Work out the finished part from the listing and answer in its coordinate system (mm). A direction names the side the tool comes from. Give positions to 0.01 mm unless a question says otherwise; leave off trailing zeros. Write each loop counter-clockwise with the first axis right and the second up, starting at its lowest first coordinate (ties: lowest second). Pieces come first, ordered by that corner, then holes. Notation, with made-up numbers: (52, -14.75) -> (57, -14.75) arc R30 ccw to (57, 24.25) -> close; hole circle Ø10 at (27.5, -5.5). An arc over 180 degrees is marked (long way). Use a Markdown table: item, result. Add a question column.
Q1. Section C-C, the plane y = 18.5 is taken. Give the vertices of the cut face in (x, z), plus the area to 3 significant figures.
Q2. Section B-B, the plane y = 33 is taken. Give the vertices of the cut face in (x, z), plus the area to 3 significant figures.
Q3. For a pull along X with two mould halves and no side action, classify faces 5 (the face through (5.4, 31.75, 0.1)), 6 (the face through (-1, 12.7, 0)), 7 (the face through (4.89, 35, 0)) as pulls with the +X half, pulls with the -X half, needs draft (parallel to the pull), parting line crosses it, or undercut.
Q4. Section A-A, the plane y = 9.5 is taken. Give the vertices of the cut face in (x, z).
Q5. Consider line 1 (Y direction, x = 7.45, z = 0); line 2 (Y direction, x = 2.75, z = 3.5); line 3 (Z direction, x = 8.45, y = 6.35). Determine where each line is inside the solid, lowest interval first.
Q6. Each of these flat-tipped pins is pushed along its axis until it touches: pin 1 Ø1.5 at (x, z) = (7, 3.5) entering from +Y; pin 2 Ø0.7 at (x, z) = (5.5, 2) entering from +Y; pin 3 Ø1 at (x, y) = (1, 18) entering from -Z; pin 4 Ø1.5 at (y, z) = (33.5, -7.5) entering from -X. Where does it stop, or does it pass through?
Q7. For faces 1 (the face through (-6.233, 28.717, 0.818)), 2 (the face through (7.14, 7.53, -0.15)), 3 (the face through (0, 38.1, 0)), 4 (the face through (4.89, 8, 0)), determine the directions among +Z, -Z, +X, -X, +Y, -Y from which every point of the face is accessible in a straight line to the end or side of a thin tool.
from build123d import *

# Parameters (mm, degrees)
SKETCH1_R           = 6.2865
BASE_EXTRUDE_DEPTH  = 38.1
SKETCH3_R           = 9.4615
BOSS_EXTRUDE1_DEPTH = 15.875
CUT_EXTRUDE1_DEPTH  = 12.7
FILLET1_R           = 4.7625
FILLET2_R           = 4.7625
SKETCH5_R           = 1.190625
CUT_EXTRUDE2_DEPTH  = 42.798101456
CUT_EXTRUDE3_START  = -6.35
CUT_EXTRUDE3_DEPTH  = 6.35
CHAMFER1_SIZE       = 0.79375


with BuildPart() as part:
    # Sketch1 → Base-Extrude (new body)
    with BuildSketch(Plane(origin=(0, 0, 0), x_dir=(-1, 0, 0), z_dir=(0, 1, 0))):
        with Locations(Location((0, 0, 0), (0, 0, 270))):
            Circle(SKETCH1_R)
    extrude(amount=BASE_EXTRUDE_DEPTH)

    # Sketch3 → Boss-Extrude1 (add)
    with BuildSketch(Plane(origin=(0, 0, 0), x_dir=(-1, 0, 0), z_dir=(0, 1, 0))):
        with Locations(Location((0, 0, 0), (0, 0, 90))):
            Circle(SKETCH3_R)
    extrude(amount=BOSS_EXTRUDE1_DEPTH)

    # Sketch4 → Cut-Extrude1 (cut)
    with BuildSketch(Plane(origin=(0, 0, 0), x_dir=(-1, 0, 0), z_dir=(0, 1, 0))):
        with BuildLine():
            Line((-4.8895, 4.247860491), (-4.8895, -4.247860491))
            ThreePointArc((-4.8895, -4.247860491), (6.477, 0), (-4.8895, 4.247860491))
        make_face()
    extrude(amount=CUT_EXTRUDE1_DEPTH, mode=Mode.SUBTRACT)

    # Fillet1
    # the kernel refuses this fillet: 4.7625 mm, written as the material it adds along each edge
    with BuildSketch(Plane(origin=(0, 15.875, 0), x_dir=(0, 0, -1), z_dir=(-1, 0, 0))) as fillet1_piece_1:
        with BuildLine():
            CenterArc((11.049, -4.490128061), FILLET1_R, 109.471220634, 70.528779366)
            Line((6.2865, -4.490128061), (6.19125, -4.490128061))
            Line((6.19125, -4.490128061), (6.19125, 0))
            Line((6.19125, 0), (6.2865, 0.09525))
            ThreePointArc((6.2865, 0.09525), (7.874, 0.09525), (9.42975, 0.089802561))
            Line((9.42975, 0.089802561), (9.4615, 0))
        make_face()
    revolve(axis=Axis((0, 15.875, 0), (0, -1, 0)))

    # Fillet2
    fillet2_edges = [part.edges().sort_by_distance(p)[0] for p in [
        (9.4615, 15.875, 0),
    ]]
    fillet(fillet2_edges, radius=FILLET2_R)

    # Sketch5 → Cut-Extrude2 (cut, through all)
    with BuildSketch(Plane.ZY.offset(-4.8895)):
        with Locations((0, 6.35)):
            Circle(SKETCH5_R)
    extrude(amount=-CUT_EXTRUDE2_DEPTH, mode=Mode.SUBTRACT)

    # Sketch7 → Cut-Extrude3 (cut)
    with BuildSketch(Plane(origin=(0, 38.1, 0), x_dir=(-1, 0, 0), z_dir=(0, 1, 0)).offset(CUT_EXTRUDE3_START)):
        with BuildLine():
            Line((-4.8895, 3.951312693), (-4.8895, -3.951312693))
            ThreePointArc((-4.8895, -3.951312693), (-6.2865, 0), (-4.8895, 3.951312693))
        make_face()
    extrude(amount=CUT_EXTRUDE3_DEPTH, mode=Mode.SUBTRACT)

    # Chamfer1
    chamfer1_edges = [part.edges().sort_by_distance(p)[0] for p in [
        (-5.67274226, 38.1, 2.70925774),
    ]]
    chamfer(chamfer1_edges, length=CHAMFER1_SIZE)


solid = part.part
Result set:
| question | item | result |
|---|---|---|
| 1 | outline | circle Ø13.33 at (0, 0) |
| 1 | area | 140 mm2 |
| 2 | outline | (4.89, -3.95) -> (4.89, 3.95) arc R6.29 ccw (long way) to start |
| 2 | area | 117 mm2 |
| 3 | face 5 | needs draft |
| 3 | face 6 | undercut |
| 3 | face 7 | pulls with the +X half |
| 4 | outline | circle Ø18.92 at (0, 0); hole (4.89, -4.25) -> (4.89, 4.25) arc R6.48 ccw (long way) to start |
| 5 | line 1 | y = 0 to 5.16, 7.54 to 17.25 |
| 5 | line 2 | y = 12.7 to 38.1 |
| 5 | line 3 | z = -4.26 to -1.19, 1.19 to 4.26 |
| 6 | pin 1 | stops at y = 17.74 |
| 6 | pin 2 | stops at y = 31.75 |
| 6 | pin 3 | stops at z = -7.18 |
| 6 | pin 4 | passes through |
| 7 | face 1 | +Y |
| 7 | face 2 | +X |
| 7 | face 3 | +Z, -Z, +X, -X, +Y |
| 7 | face 4 | -Y |
